Verification items for the finished model (mm, model axes). A direction names the side the tool comes from. Give positions to 0.01 mm unless a question says otherwise; leave off trailing zeros. Loops run counter-clockwise (first coordinate to the right, second up) from the corner with the lowest first, then second, coordinate; pieces in that order, holes last. Notation, with made-up numbers: (8.25, 48) - (17.25, 48) arc R19 cw to (17.25, 64) - close; hole circle Ø11 at (55.25, -10). An arc over 180 degrees is marked (long way). One line per item, written item: value. Start each with the question number.
1. Access from +Z, -Z, +X, -X, +Y, -Y to the whole of each face (thin tool, end or side, straight path). Record for faces 4 (the cylindrical face through (17.26, -61.81, 69.17)), 5 (the flat face through (13, 13, 78.5)), 6 (the flat face through (35, 24.1, -71.5)).
2. Mould release check, pull along X, two halves, no side actions. Record for faces 1 (the flat face through (0, -1, -1)), 2 (the cylindrical face through (14.5, 7.96, 79.24)), 3 (the cylindrical face through (17.255, 70.125, 66.138)): pulls with the +X half, pulls with the -X half, needs draft (parallel to the pull), parting line crosses it, or undercut.
3. Sectioned sample at B-B (x = 53). Record the cut outline in (y, z), plus the area to 3 significant figures.
4. Gauge pin test, flat ends, axial feed: pin 1 (10 mm diameter, centred on x = 43.5, z = -57.5, fed in from -Y); pin 2 (7 mm diameter, centred on y = 17.5, z = 50, fed in from +X). Record the tip position at first contact, or that the pin passes through.
5. Scan lines: L1, parallel to Z at x = 11.5, y = -65; L2, parallel to Y at x = 17, z = 65. Record each from-to range of solid material in increasing order. Write a range as [from, to].
6. Sectioned sample at A-A (z = 0). Record the cut outline in (x, y), plus the area to 3 significant figures.
Autodesk Inventor part; units mm, degrees
ref_plane "YZ Plane" through (0, 0, 0) normal (1, 0, 0) x (0, 1, 0)
ref_plane "XZ Plane" through (0, 0, 0) normal (0, 1, 0) x (-1, 0, 0)
ref_plane "XY Plane" through (0, 0, 0) normal (0, 0, 1) x (1, 0, 0)
sketch "Skizze1" plane through (0, 0, 0) normal (0, 0, 1) x (1, 0, 0)
  line L0 (0, 80) -> (35, 80)
  line L1 (35, 80) -> (35, -80)
  line L2 (35, -80) -> (0, -80)
  line L3 (0, -80) -> (0, 80)
  line L4 (35, 75) -> (57.5, 75)
  line L5 (57.5, 75) -> (57.5, 0)
  line L6 (57.5, 0) -> (35, 0)
  line L7 (35, 0) -> (35, 75)
  point P0 (0, 0)
  point P1 (0, 0)
  dimension "d0" = 160
  dimension "d1" = 150
  dimension "d2" = 57.5
  dimension "d3" = 35
extrude "Extrusion1" add sketch "Skizze1" along normal mid plane 160 contours L0 L1 L2 L3
revolve "Umdrehung1" add sketch "Skizze1" angle 360 about axis through (57.5, 0, 0) along (-1, 0, 0) contours L4 L5 L6 L1
fillet "Rundung1" radius 15 4 edges at (17.5, 80, 80) (17.5, 80, -80) (17.5, -80, 80) (17.5, -80, -80)
sketch "Skizze2" plane through (35, -65, -80) normal (1, 0, 0) x (0, 0, -1)
  line L0 (-15, 0) -> (-145, 0)
  line L1 (-145, 0) -> (-145, 130)
  line L2 (-145, 130) -> (-15, 130)
  line L3 (-15, 130) -> (-15, 0)
  line L4 (-15, 0) -> (-145, 130) construction
  line L5 (-145, 0) -> (-15, 130) construction
  point P0 (-80, 65)
  dimension "d8" = 130
  dimension "d9" = 130
hole "Bohrung1" at (35, 65, 65) at (35, 65, -65) at (35, -65, 65) at (35, -65, -65) direction (-1, 0, 0) diameter 10.5 end through all
sketch "Skizze3" plane through (0, 0, 80) normal (0, 0, 1) x (1, 0, 0)
  line L0 (35, 80) -> (0, 80)
  line L1 (0, 65) -> (0, -65)
  point P0 (0, 0)
  point P1 (17.5, 17.5)
  dimension "d17" = 62.5
  dimension "d18" = 17.5
hole "Bohrung2" at (17.5, 17.5, 80) direction (0, 0, -1) diameter 8.376 depth 34.5 tip angle 118 counterbore diameter 20 counterbore depth 1.5
sketch "Skizze4" plane through (57.5, 0, 0) normal (1, 0, 0) x (0, 0, -1)
  line L0 (-80, -65) -> (-80, 65)
  line L1 (65, 80) -> (-65, 80)
  point P0 (0, 0)
  point P1 (-50, 17.5)
  dimension "d26" = 30
  dimension "d27" = 62.5
hole "Bohrung3" at (57.5, 17.5, 50) direction (-1, 0, 0) diameter 8.5 depth 40 tip angle 118
chamfer "Fase1" distance 2 angle 45 1 edges at (17.5, 21.688, 78.5)
chamfer "Fase2" distance 1.5 angle 45 1 edges at (57.5, -75, 0)
equation "\"d4\" = d0"
properties part number "Deckel_hinten" material "Stahl AISI 4130"
Results are:
1. face 4: +X, -X
1. face 5: +Z
1. face 6: +X
2. face 1: pulls with the -X half
2. face 2: undercut
2. face 3: needs draft
3. outline: circle Ø150 at (0, 0); hole circle Ø8.5 at (17.5, 50)
3. area: 17,600 mm^2
4. pin 1: stops at y = -53.56
4. pin 2: stops at x = 15.2
5. L1: z = [-80, -70.25], [-59.75, 59.75], [70.25, 80]
5. L2: y = [-80, -70.25], [-59.75, 13.34], [21.66, 59.75], [70.25, 80]
6. outline: (0, -80) - (35, -80) - (35, -75) - (56, -75) - (57.5, -73.5) - (57.5, 73.5) - (56, 75) - (35, 75) - (35, 80) - (0, 80) - close
6. area: 8,970 mm^2
